Design review of the part built by this model. Coordinates are the model's own, in mm. Face numbers are marked on the shaded views. Coordinates: 2 decimals unless noted, no trailing zeros. Loops run counter-clockwise (first coordinate to the right, second up) from the corner with the lowest first, then second, coordinate; pieces in that order, holes last.
Q1. Add section A-A on x = -5.5. Give the boundary of the cut face in (y, z), and give its area (3 significant figures).
Q2. Add section D-D on z = 1.4. Give the number of separate pieces and of enclosed holes in the cut face, and give its area (3 significant figures).
Q3. Wall thickness on probe 1 along Y at (x, z) = (-0.5, 2.05); probe 2 along X at (y, z) = (11, 1.25); probe 3 along Y at (x, z) = (-7.5, 0.4): over which ranges is each line inside the solid? List them lowest first.
Q4. Draft analysis for pull direction Z (two halves, no side actions). For the marked faces 1 and 2, state which applies: released by +Z, released by -Z, zero draft, split by the parting line, or undercut.
Q5. Add section C-C on x = 1. Give the boundary of the cut face in (y, z).
Q6. For P1, Ø8.5, axis at x = 0.31, y = 9.15, coming from the +Z side, flat-tipped, find the tip position at first contact; note if it passes through.
Q7. Add section B-B on y = -56. Give the boundary of the cut face in (x, z), and give its area (3 significant figures).
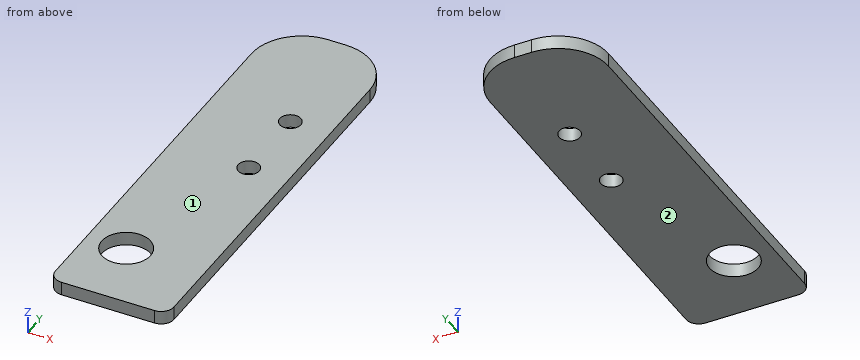
Autodesk Inventor part; units mm, degrees
ref_plane "YZ Plane" through (0, 0, 0) normal (1, 0, 0) x (0, 1, 0)
ref_plane "XZ Plane" through (0, 0, 0) normal (0, 1, 0) x (-1, 0, 0)
ref_plane "XY Plane" through (0, 0, 0) normal (0, 0, 1) x (1, 0, 0)
sketch "Sketch1" plane through (0, 0, 0) normal (0, 0, 1) x (1, 0, 0)
  line L0 (-19.4806, -69.0981) -> (-16.0643, -69.0981)
  line L1 (-16.0643, 40.9019) -> (-19.4806, 40.9019)
  circle A0 centre (0.3057, -10.8501) radius 2.65
  circle A1 centre (0.3057, 9.1499) radius 2.65
  line L2 (-19.4806, -64.0981) -> (-19.4806, 35.9019)
  line L3 (60.4357, -17.8501) -> (60.4357, 16.1499)
  arc A2 (32.4357, 9.8999) -> (32.4357, -11.6001) centre (32.4357, -0.8501) ccw
  circle A3 centre (-9.5643, -50.8501) radius 6.125
  line L4 (10.3057, 75.9749) -> (10.3057, -77.6751)
  line L5 (-19.4806, -69.0981) -> (10.3057, -69.0981)
  line L6 (10.3057, -69.0981) -> (10.3057, 40.9019)
  line L7 (10.3057, 40.9019) -> (-19.4806, 40.9019)
  line L8 (-19.4806, 40.9019) -> (-19.4806, -69.0981)
  point P0 (0, 0)
extrude "Extrusion1" add sketch "Sketch1" along normal blind 3.4163
fillet "Fillet1" radius 3.175 2 edges at (10.3057, -69.0981, 1.7082) (-19.4806, -69.0981, 1.7082)
fillet "Fillet2" radius 12.7 2 edges at (-19.4806, 40.9019, 1.7082) (10.3057, 40.9019, 1.7082)
properties part number "z_screw_bottom_mount" material "Steel, Mild"
Entries:
1. outline: (-69.1, 0) - (-55.43, 0) - (-55.43, 3.42) - (-69.1, 3.42) - close; (-46.27, 0) - (40.9, 0) - (40.9, 3.42) - (-46.27, 3.42) - close
1. area: 344 mm2
2. separate pieces: 1
2. enclosed holes: 3
2. area: 3,040 mm2
3. probe 1: y = -69.1 to -13.37, -8.33 to 6.63, 11.67 to 40.76
3. probe 2: x = -19.48 to -1.59, 2.2 to 10.31
3. probe 3: y = -69.1 to -56.62, -45.08 to 40.88
4. face 1: released by +Z
4. face 2: released by -Z
5. outline: (-69.1, 0) - (-13.41, 0) - (-13.41, 3.42) - (-69.1, 3.42) - close; (-8.29, 0) - (6.59, 0) - (6.59, 3.42) - (-8.29, 3.42) - close; (11.71, 0) - (40.44, 0) - (40.44, 3.42) - (11.71, 3.42) - close
6. P1: stops at z = 3.42
7. outline: (-19.48, 0) - (-12.88, 0) - (-12.88, 3.42) - (-19.48, 3.42) - close; (-6.25, 0) - (10.31, 0) - (10.31, 3.42) - (-6.25, 3.42) - close
7. area: 79.1 mm2
